Geometry: see drawing. Coordinates: mm, zero at the bounding-box minimum. Round coordinates to 2 decimals unless told otherwise and drop trailing zeros. Loops run counter-clockwise (first coordinate to the right, second up) from the corner with the lowest first, then second, coordinate; pieces in that order, holes last. Notation, with made-up numbers: (-32.5, -20.75) - (2.5, -20.75) arc R17 cw to (2.5, -8.75) - close; hole circle Ø10 at (75.5, 26.5). An arc over 180 degrees is marked (long way). Answer in a Markdown table with one row per item. Add a question column.
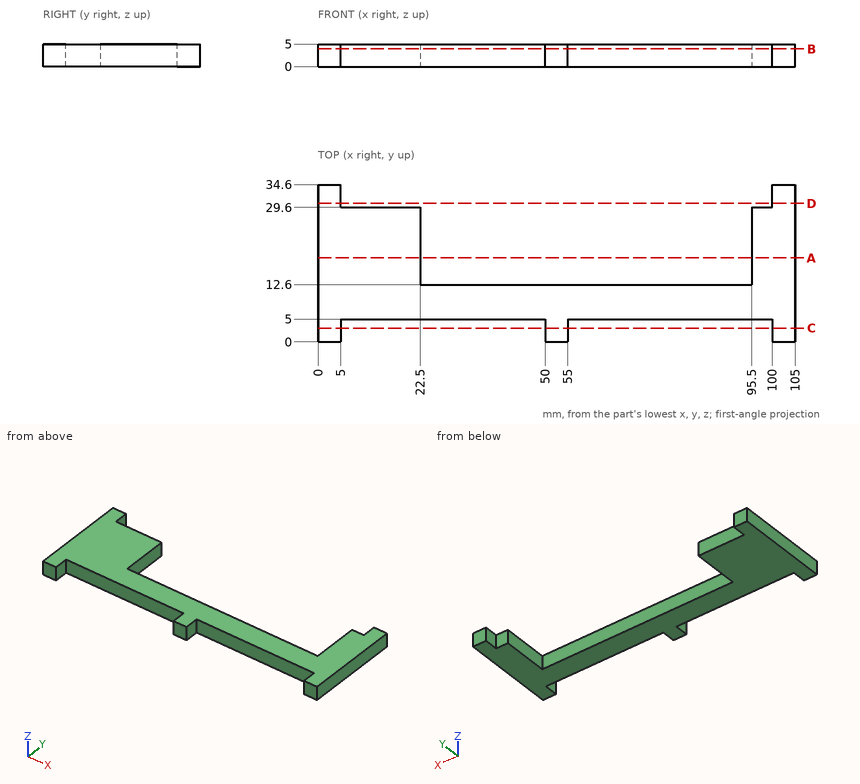
1) Section A-A, the plane y = 18.5. Return the cut outline in (x, z), and give its area (3 significant figures).
2) Contact query for flat-ended pins moving along their axis: pin 1 Ø3 at (x, z) = (36.5, 0.5) entering from -Y; pin 2 Ø1.5 at (x, z) = (80.5, 2.5) entering from +Y. Output: stop coordinate, or through.
3) Section D-D, the plane y = 30.5. Return the cut outline in (x, z), and give its area (3 significant figures).
4) Material intervals for line 1 along X through (y, z) = (4.5, 3.95); line 2 along X through (y, z) = (16.5, 1.4); line 3 along Y through (x, z) = (35, 0.5), sorted ascending. Write a range as from..to.
5) Section B-B, the plane z = 3.95. Return the cut outline in (x, y).
6) Section C-C, the plane y = 3. Return the cut outline in (x, z).
Evaluation:
| question | item | result |
|---|---|---|
| 1 | outline | (0, 0) - (22.5, 0) - (22.5, 5) - (0, 5) - close; (95.5, 0) - (105, 0) - (105, 5) - (95.5, 5) - close |
| 1 | area | 160 mm² |
| 2 | pin 1 | stops at y = 5 |
| 2 | pin 2 | stops at y = 12.6 |
| 3 | outline | (0, 0) - (5, 0) - (5, 5) - (0, 5) - close; (100, 0) - (105, 0) - (105, 5) - (100, 5) - close |
| 3 | area | 50.0 mm² |
| 4 | line 1 | x = 0..5, 50..55, 100..105 |
| 4 | line 2 | x = 0..22.5, 95.5..105 |
| 4 | line 3 | y = 5..12.6 |
| 5 | outline | (0, 0) - (5, 0) - (5, 5) - (50, 5) - (50, 0) - (55, 0) - (55, 5) - (100, 5) - (100, 0) - (105, 0) - (105, 34.6) - (100, 34.6) - (100, 29.6) - (95.5, 29.6) - (95.5, 12.6) - (22.5, 12.6) - (22.5, 29.6) - (5, 29.6) - (5, 34.6) - (0, 34.6) - close |
| 6 | outline | (0, 0) - (5, 0) - (5, 5) - (0, 5) - close; (50, 0) - (55, 0) - (55, 5) - (50, 5) - close; (100, 0) - (105, 0) - (105, 5) - (100, 5) - close |
